For this review, take the finished solid that the model builds, in its own axes (mm). Round coordinates to 2 decimals unless told otherwise and drop trailing zeros. Loops run counter-clockwise (first coordinate to the right, second up) from the corner with the lowest first, then second, coordinate; pieces in that order, holes last. Notation, with made-up numbers: (73, 40) -> (99, 40) arc R23 cw to (99, 61) -> close; hole circle Ø10 at (58, 39). An arc over 180 degrees is marked (long way). Write each question's results on one line, items separated by ' | '.
```python
from build123d import *

# Parameters (mm, degrees)
BOSS_EXTRUDE1_DEPTH = 2.54
SKETCH4_R           = 2.0955
CUT_EXTRUDE2_DEPTH  = 121.080498


with BuildPart() as part:
    # Sketch1 → Boss-Extrude1 (new body)
    with BuildSketch(Plane(origin=(0, 0, 0), x_dir=(1, 0, 0), z_dir=(0, 1, 0))):
        with BuildLine():
            Line((0, 0), (-119.38, 0))
            Line((-119.38, 0), (-119.38, 12.7))
            Line((-119.38, 12.7), (9.042090255, 12.7))
            ThreePointArc((9.042090255, 12.7), (11.44680364, 10.977895798), (10.590755588, 8.146735068))
            Line((10.590755588, 8.146735068), (0, 0))
        make_face()
    extrude(amount=BOSS_EXTRUDE1_DEPTH)

    # Sketch4 → Cut-Extrude2 (cut, through all)
    with BuildSketch(Plane(origin=(0, 2.54, 0), x_dir=(1, 0, 0), z_dir=(0, 1, 0))):
        with Locations(Location((-113.03, 6.35, 0), (0, 0, 270))):
            Circle(SKETCH4_R)
    extrude(amount=-CUT_EXTRUDE2_DEPTH, mode=Mode.SUBTRACT)


solid = part.part
```
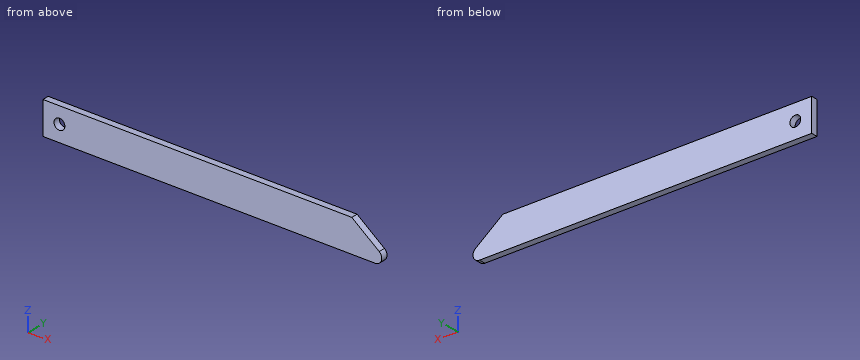
1. Consider section A-A (x = -113.03). State the section outline as (y, z) points.
Values found:
outline: (0, -12.7) -> (2.54, -12.7) -> (2.54, -8.45) -> (0, -8.45) -> close; (0, -4.25) -> (2.54, -4.25) -> (2.54, 0) -> (0, 0) -> close
2. Consider section B-B (y = 1.1). State the section outline as (x, z) points, plus the area to 3 significant figures.
Values found:
outline: (-119.38, -12.7) -> (9.04, -12.7) arc R2.54 ccw to (10.59, -8.15) -> (0, 0) -> (-119.38, 0) -> close; hole circle Ø4.19 at (-113.03, -6.35) | area: 1,600 mm2
3. To check wall thickness, follow probe 1 along X at (y, z) = (0.85, -6.5); probe 2 along X at (y, z) = (1.55, -8); probe 3 along X at (y, z) = (2, -10.75). State the ranges of each line that lie inside material, in increasing order.
Values found:
probe 1: x = -119.38 to -115.12, -110.94 to 8.45 | probe 2: x = -119.38 to -114.32, -111.74 to 10.4 | probe 3: x = -119.38 to 11.51
4. Consider section D-D (z = -1.25). State the section outline as (x, y) points (3 decimals).
Values found:
outline: (-119.38, 0) -> (1.625, 0) -> (1.625, 2.54) -> (-119.38, 2.54) -> close
5. Consider section C-C (z = -6.35). State the section outline as (x, y) points (1 decimal), plus the area to 3 significant figures.
Values found:
outline: (-119.4, 0) -> (-115.1, 0) -> (-115.1, 2.5) -> (-119.4, 2.5) -> close; (-110.9, 0) -> (8.3, 0) -> (8.3, 2.5) -> (-110.9, 2.5) -> close | area: 314 mm2
